For this review, take the finished solid that the model builds, in its own axes (mm). A direction names the side the tool comes from. Coordinates: 2 decimals unless noted, no trailing zeros. Loops run counter-clockwise (first coordinate to the right, second up) from the corner with the lowest first, then second, coordinate; pieces in that order, holes last. Notation, with made-up numbers: M 2,60.25 L 53,60.25 A31 cw 53,86.25 Z; hole C 17,40.5 d7. An arc over 180 degrees is marked long. Use one line per item in the form item = value.
```python
from build123d import *

# Parameters (mm, degrees)
BOSS_EXTRUDE1_DEPTH      = 10
BOSS_EXTRUDE2_DEPTH      = 40
BOSS_EXTRUDE2_DEPTH_BACK = 10
SKETCH2_W                = 50
SKETCH2_H                = 10
SKETCH3_R                = 25
BOSS_EXTRUDE3_DEPTH      = 10
BOSS_EXTRUDE4_START      = -10
SKETCH4_R                = 25
BOSS_EXTRUDE4_DEPTH      = 10
CUT_EXTRUDE1_START       = -40
SKETCH5_R                = 15
CUT_EXTRUDE1_DEPTH       = 40


with BuildPart() as part:
    # Sketch1 → Boss-Extrude1 (new body)
    with BuildSketch(Plane(origin=(0, 0, 0), x_dir=(1, 0, 0), z_dir=(0, 1, 0))):
        with BuildLine():
            Line((15, 20), (-65, 20))
            ThreePointArc((-65, 20), (-85, 0), (-65, -20))
            Line((-65, -20), (15, -20))
            Line((15, -20), (15, -10))
            Line((15, -10), (65, -10))
            Line((65, -10), (65, 10))
            Line((65, 10), (15, 10))
            Line((15, 10), (15, 20))
        make_face()
        with BuildLine():
            ThreePointArc((-25, 10), (-15, 0), (-25, -10))
            Line((-25, -10), (-65, -10))
            ThreePointArc((-65, -10), (-75, 0), (-65, 10))
            Line((-65, 10), (-25, 10))
        make_face(mode=Mode.SUBTRACT)
    extrude(amount=BOSS_EXTRUDE1_DEPTH)

    # Sketch2 → Boss-Extrude2 (add, two sides: drawn at the far end of the back side and taken through both)
    with BuildSketch(Plane(origin=(0, 10, 0), x_dir=(1, 0, 0), z_dir=(0, 1, 0)).offset(-BOSS_EXTRUDE2_DEPTH_BACK)):
        with Locations((40, -15)):
            Rectangle(SKETCH2_W, SKETCH2_H)
        with Locations((40, 15)):
            Rectangle(SKETCH2_W, SKETCH2_H)
    extrude(amount=BOSS_EXTRUDE2_DEPTH + BOSS_EXTRUDE2_DEPTH_BACK)

    # Sketch3 → Boss-Extrude3 (add)
    with BuildSketch(Plane.XY.offset(20)):
        with Locations((40, 50)):
            Circle(SKETCH3_R)
    extrude(amount=-BOSS_EXTRUDE3_DEPTH)

    # Sketch4 → Boss-Extrude4 (add)
    with BuildSketch(Plane(origin=(0, 0, -20), x_dir=(-1, 0, 0), z_dir=(0, 0, -1)).offset(BOSS_EXTRUDE4_START)):
        with Locations((-40, 50)):
            Circle(SKETCH4_R)
    extrude(amount=BOSS_EXTRUDE4_DEPTH)

    # Sketch5 → Cut-Extrude1 (cut)
    with BuildSketch(Plane.XY.offset(20).offset(CUT_EXTRUDE1_START)):
        with Locations((40, 50)):
            Circle(SKETCH5_R)
    extrude(amount=CUT_EXTRUDE1_DEPTH, mode=Mode.SUBTRACT)


solid = part.part
```
1. Consider section B-B on x = -51. Write out the cut boundary in (y, z).
Computed values:
outline = M 0,-20 L 10,-20 L 10,-10 L 0,-10 Z; M 0,10 L 10,10 L 10,20 L 0,20 Z
2. Consider section A-A on z = 0. Write out the cut boundary in (x, y).
Computed values:
outline = M -85,0 L -75,0 L -75,10 L -85,10 Z; M -15,0 L 65,0 L 65,10 L -15,10 Z
3. Consider section D-D on y = 62. Write out the cut boundary in (x, z).
Computed values:
outline = M 18.07,-20 L 31,-20 L 31,-10 L 18.07,-10 Z; M 18.07,10 L 31,10 L 31,20 L 18.07,20 Z; M 49,-20 L 61.93,-20 L 61.93,-10 L 49,-10 Z; M 49,10 L 61.93,10 L 61.93,20 L 49,20 Z
4. Tool access review of faces 4 (the face through (-75, 5, 0)), 5 (the face through (34, 36, 10)), 6 (the face through (15, 30, -15)): name each direction out of +Z, -Z, +X, -X, +Y, -Y from which nothing blocks a thin tool from reaching the whole face with its end or side.
Computed values:
face_4 = +Y, -Y
face_5 = +X, -X, +Y
face_6 = +Z, -Z, -X, +Y
5. Consider section C-C on x = 40. Write out the cut boundary in (y, z), plus the area to 3 significant figures.
Computed values:
outline = M 0,-20 L 35,-20 L 35,-10 L 10,-10 L 10,10 L 35,10 L 35,20 L 0,20 Z; M 65,-20 L 75,-20 L 75,-10 L 65,-10 Z; M 65,10 L 75,10 L 75,20 L 65,20 Z
area = 1,100 mm2
6. Wall thickness on line 1 along Y through (x, z) = (40, 16); line 2 along Z through (x, y) = (35.5, 23); line 3 along X through (y, z) = (50, 15.25): over which ranges is each line inside the solid? List them lowest first. Write a range as from..to.
Computed values:
line_1 = 0..35, 65..75
line_2 = -20..-10, 10..20
line_3 = 15..25, 55..65
7. For pin 1 Ø5 at (y, z) = (26.5, -16) entering from -X; pin 2 Ø24 at (x, y) = (40, 50) entering from +Z; pin 3 Ø1.5 at (y, z) = (67, 11.5) entering from -X; pin 4 Ø4 at (x, z) = (25.5, -6.5) entering from +Y, all flat-tipped, find the tip position at first contact; note any pin that passes through.
Computed values:
pin_1 = 15
pin_2 = through
pin_3 = 21
pin_4 = 10
8. Draft analysis for pull direction X (two halves, no side actions). For faces 1 (the face through (-11, 10, 0)), 2 (the face through (-45, 5, -10)), 3 (the face through (-85, 5, 0)), state which applies: +X half, -X half, draft (parallel to the pull), parting line (faces both ways), or undercut.
Computed values:
face_1 = draft
face_2 = undercut
face_3 = -X half
